Geometry: final body of the model. Coordinates: model frame, mm. Face numbers are marked on the shaded views. A direction names the side the tool comes from. Round coordinates to 2 decimals unless told otherwise and drop trailing zeros. Order: outer loops, then holes, each group sorted by start corner. A loop starts at its lowest first (then second) coordinate and runs counter-clockwise, first axis right, second up. Notation, with made-up numbers: M 50.25,-6.75 L 80.25,-6.75 A23 cw 80.25,7.25 Z; hole C 4,-1 d1. An arc over 180 degrees is marked long. Return JSON: item names as keys, results as strings. Group by question number.
Q1. Ray query, probe 1 along X at (y, z) = (-13.5, 17.5); probe 2 along Z at (x, y) = (-10, -18); probe 3 along Y at (x, z) = (44.5, 19). Return the intervals inside material, ascending.
Q2. Cut plane C-C on x = 41.5. Output: boundary loops of the cut face in (y, z), and give its area (3 significant figures).
Q3. Access query for the marked faces 5, 6 and 7. Directions: +Z, -Z, +X, -X, +Y, -Y. A direction counts if a zero-diameter tool reaches every point of the face in a straight line with its end or side. Return the directions, or none.
Q4. Cut plane D-D on y = 50. Output: boundary loops of the cut face in (x, z).
Q5. Cut plane A-A on z = -2. Output: boundary loops of the cut face in (x, y).
Q6. Mould query, pull axis Z, two halves, no side actions, for the marked faces 1, 2, 3 and 4. Classes: released by +Z, released by -Z, zero draft, split by the parting line, or undercut.
Q7. Cut plane B-B on y = -31.5. Output: boundary loops of the cut face in (x, z), and give its area (3 significant figures).
```python
from build123d import *

# Parameters (mm, degrees)
F0_W     = 50
F0_H     = 50
F0_W_2   = 46
F0_H_2   = 46
F1_DEPTH = 75
F2_W     = 70
F2_H     = 50
F2_W_2   = 66
F2_H_2   = 46
F3_DEPTH = 35


with BuildPart() as f1:
    # F0 (on Front) → F1 (new body, symmetric)
    with BuildSketch(Plane.XZ):
        Rectangle(F0_W, F0_H)
        Rectangle(F0_W_2, F0_H_2, mode=Mode.SUBTRACT)
    extrude(amount=F1_DEPTH, both=True)

    # F2 (on face) → F3 (join)
    with BuildSketch(Plane.YZ.offset(25)):
        with Locations((40, 0)):
            Rectangle(F2_W, F2_H)
        with Locations((40, 0)):
            Rectangle(F2_W_2, F2_H_2, mode=Mode.SUBTRACT)
    extrude(amount=F3_DEPTH)

    # F5: F1 across plane


with BuildPart() as f1_1:
    add(f1.part)
    add(f1.part.mirror(Plane(origin=(60, 40, 0), x_dir=(0, 1, 0), z_dir=(1, 0, 0))))


solid = f1_1.part
```
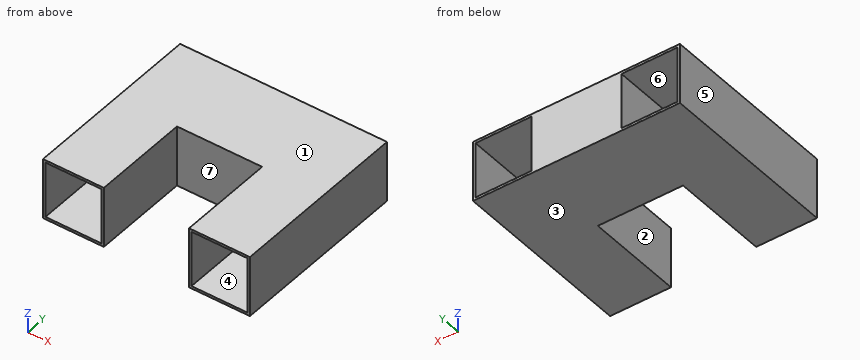
Result sheet:
{
 "1": {"probe 1": "x = -25 to -23, 23 to 25, 95 to 97, 143 to 145", "probe 2": "z = -25 to -23, 23 to 25", "probe 3": "y = 5 to 7, 73 to 75"},
 "2": {"outline": "M 5,-25 L 75,-25 L 75,25 L 5,25 Z; hole M 7,-23 L 73,-23 L 73,23 L 7,23 Z", "area": "464 mm²"},
 "3": {"face 5": "+Z, -Z, -X, +Y, -Y", "face 6": "+Y, -Y", "face 7": "+Z, -Z, -Y"},
 "4": {"outline": "M -25,-25 L 145,-25 L 145,25 L -25,25 Z; hole M -23,-23 L 23,-23 L 23,23 L -23,23 Z; hole M 25,-23 L 95,-23 L 95,23 L 25,23 Z; hole M 97,-23 L 143,-23 L 143,23 L 97,23 Z"},
 "5": {"outline": "M -25,-75 L -23,-75 L -23,75 L -25,75 Z; M 23,-75 L 25,-75 L 25,5 L 95,5 L 95,-75 L 97,-75 L 97,75 L 23,75 Z; M 143,-75 L 145,-75 L 145,75 L 143,75 Z; hole M 25,7 L 95,7 L 95,73 L 25,73 Z"},
 "6": {"face 1": "released by +Z", "face 2": "zero draft", "face 3": "released by -Z", "face 4": "undercut"},
 "7": {"outline": "M -25,-25 L 25,-25 L 25,25 L -25,25 Z; M 95,-25 L 145,-25 L 145,25 L 95,25 Z; hole M -23,-23 L 23,-23 L 23,23 L -23,23 Z; hole M 97,-23 L 143,-23 L 143,23 L 97,23 Z", "area": "768 mm²"}
}
